For this review, take the finished solid that the model builds, in its own axes (mm). Face numbers are marked on the shaded views. A direction names the side the tool comes from. Coordinates: 2 decimals unless noted, no trailing zeros. Write each loop counter-clockwise with the first axis right and the second up, starting at its lowest first coordinate (ties: lowest second). Pieces come first, ordered by that corner, then holes. Notation, with made-up numbers: (4.25, -11.5) - (20.25, -11.5) arc R22 cw to (20.25, 24.5) - close; hole circle Ø4 at (1, -28.75). An arc over 180 degrees is marked (long way). Write each question's results on one line, items separated by ' | '.
from build123d import *

# Parameters (mm, degrees)
BOSS_EXTRUDE1_DEPTH     = 177.8
BOSS_EXTRUDE2_DEPTH     = 6.35
BOSS_EXTRUDE3_START     = -6.35
BOSS_EXTRUDE3_DEPTH     = 6.35
SKETCH5_W               = 81.82
SKETCH5_H               = 165.1
CUT_EXTRUDE1_DEPTH      = 216.897319711
BOSS_EXTRUDE6_DEPTH     = 165.1
CUT_EXTRUDE2_DEPTH      = 212.237817104
CUT_EXTRUDE2_DEPTH_BACK = 212.237817104
SKETCH9_R               = 1.4605
SKETCH10_R              = 0.2159
CUT_EXTRUDE3_DEPTH      = 212.237817104


with BuildPart() as part:
    # Sketch1 → Boss-Extrude1 (new body)
    with BuildSketch(Plane.XY):
        with BuildLine():
            Line((0, 12.912727148), (-56.568542495, 69.481269642))
            Line((-56.568542495, 69.481269642), (-61.058670555, 64.991141582))
            Line((-61.058670555, 64.991141582), (-4.490128061, 8.422599087))
            ThreePointArc((-4.490128061, 8.422599087), (5.116694028, -14.770321092), (-4.490128061, -37.96324127))
            Line((-4.490128061, -37.96324127), (-58.371664787, -91.844777996))
            Line((-58.371664787, -91.844777996), (-53.881536726, -96.334906057))
            Line((-53.881536726, -96.334906057), (0, -42.453369331))
            ThreePointArc((0, -42.453369331), (11.466694028, -14.770321092), (0, 12.912727148))
        make_face()
    extrude(amount=BOSS_EXTRUDE1_DEPTH)

    # Sketch2 → Boss-Extrude2 (add)
    with BuildSketch(Plane(origin=(0, 0, 0), x_dir=(-1, 0, 0), z_dir=(0, 0, -1))):
        with BuildLine():
            Line((61.058670555, 64.991141582), (58.371664787, -91.844777996))
            Line((58.371664787, -91.844777996), (4.490128061, -37.96324127))
            ThreePointArc((4.490128061, -37.96324127), (-5.116694028, -14.770321092), (4.490128061, 8.422599087))
            Line((4.490128061, 8.422599087), (61.058670555, 64.991141582))
        make_face()
    extrude(amount=-BOSS_EXTRUDE2_DEPTH)

    # Sketch4 → Boss-Extrude3 (add)
    with BuildSketch(Plane.XY.offset(177.8).offset(BOSS_EXTRUDE3_START)):
        with BuildLine():
            Line((-61.058670555, 64.991141582), (-58.371664787, -91.844777996))
            Line((-58.371664787, -91.844777996), (-4.490128061, -37.96324127))
            ThreePointArc((-4.490128061, -37.96324127), (5.116694028, -14.770321092), (-4.490128061, 8.422599087))
            Line((-4.490128061, 8.422599087), (-61.058670555, 64.991141582))
        make_face()
    extrude(amount=BOSS_EXTRUDE3_DEPTH)

    # Sketch5 → Cut-Extrude1 (cut, through all)
    with BuildSketch(Plane(origin=(21.226684665, -21.226684665, 0), x_dir=(0.7071067811865512, 0.7071067811865439, 0), z_dir=(0.7071067811865439, -0.7071067811865512, 0))):
        with Locations((-63.309065338, 88.9)):
            Rectangle(SKETCH5_W, SKETCH5_H)
    extrude(amount=-CUT_EXTRUDE1_DEPTH, mode=Mode.SUBTRACT)

    # Sketch8 → Boss-Extrude6 (add)
    with BuildSketch(Plane.XY.offset(6.35)):
        Polygon((-50.843145831, -78.430564434), (-46.35301777, -82.920692495), (-52.467323164, -94.920692495), (-56.957451225, -90.430564434), align=None)
    extrude(amount=BOSS_EXTRUDE6_DEPTH)

    # Sketch9 → Cut-Extrude2 (cut, two sides: drawn at the far end of the back side and taken through both)
    with BuildSketch(Plane.XY.offset(177.8).offset(-CUT_EXTRUDE2_DEPTH_BACK)):
        with Locations((-56.568542495, 51.5207574)):
            Circle(SKETCH9_R)
        with Locations((-38.608030253, 33.560245158)):
            Circle(SKETCH9_R)
    extrude(amount=CUT_EXTRUDE2_DEPTH + CUT_EXTRUDE2_DEPTH_BACK, mode=Mode.SUBTRACT)

    # Sketch10 → Cut-Extrude3 (cut, through all)
    with BuildSketch(Plane(origin=(0, 0, 0), x_dir=(-1, 0, 0), z_dir=(0, 0, -1))):
        with Locations((49.930224033, -91.305962629)):
            Circle(SKETCH10_R)
        with Locations((35.788088496, -77.163827092)):
            Circle(SKETCH10_R)
        with Locations((21.645952872, -63.021691468)):
            Circle(SKETCH10_R)
        with Locations((7.503817248, -48.879555844)):
            Circle(SKETCH10_R)
        with Locations((-6.638318376, -34.737420221)):
            Circle(SKETCH10_R)
    extrude(amount=-CUT_EXTRUDE3_DEPTH, mode=Mode.SUBTRACT)


solid = part.part
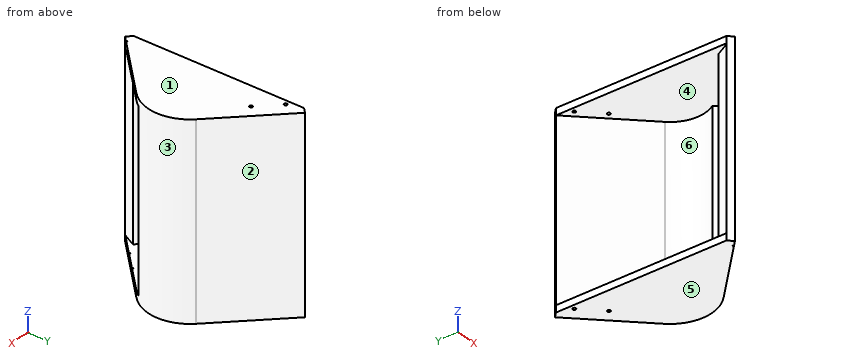
Q1. Mouldability with a two-part tool opening along Y and no side actions: class the marked faces 1, 2, 3 and 4 as pulls with the +Y half, pulls with the -Y half, needs draft (parallel to the pull), parting line crosses it, or undercut.
Results found:
face 1: needs draft | face 2: pulls with the +Y half | face 3: parting line crosses it | face 4: undercut
Q2. Wall thickness on line 1 along Z through (x, y) = (-29.5, -51.5); line 2 along Y through (x, z) = (-49, 49.5): over which ranges is each line inside the solid? List them lowest first. Write a range as from..to.
Results found:
line 1: 0..6.35, 171.45..177.8 | line 2: -88.12..-80.27, 52.93..61.91
Q3. Take a section at A-A on z = 105.5. State the section outline as (x, y) points.
Results found:
outline: (-61.06, 64.99) - (-4.49, 8.42) arc R32.8 cw to (0.26, -31.94) - (4.86, -36.54) arc R39.15 ccw to (0, 12.91) - (-56.57, 69.48) - close; (-58.37, -91.84) - (-53.88, -96.33) - (-52.47, -94.92) - (-46.35, -82.92) - (-50.84, -78.43) - (-56.96, -90.43) - close
Q4. Take a section at C-C on x = -19. State the section outline as (y, z) points, plus the area to 3 significant figures.
Results found:
outline: (-61.45, 0) - (31.91, 0) - (31.91, 177.8) - (-61.45, 177.8) - (-61.45, 171.45) - (22.93, 171.45) - (22.93, 6.35) - (-61.45, 6.35) - close | area: 2,670 mm2
Q5. For pin 1 (10 mm diameter, centred on y = -6.5, z = 44.5, fed in from +X); pin 2 (5 mm diameter, centred on y = 43.5, z = 27.5, fed in from +X); pin 3 (6 mm diameter, centred on x = -26, z = 96.5, fed in from -Y); pin 4 (2.5 mm diameter, centred on x = -38.61, y = 33.56, fed in from -Z), all flat-tipped, find the tip position at first contact; note any pin that passes through.
Results found:
pin 1: x = 11.33 | pin 2: x = -28.09 | pin 3: y = 26.93 | pin 4: through
Q6. Take a section at D-D on y = 16.5. State the section outline as (x, z) points, plus the area to 3 significant figures.
Results found:
outline: (-60.23, 0) - (-3.59, 0) - (-3.59, 177.8) - (-60.23, 177.8) - (-60.23, 171.45) - (-12.57, 171.45) - (-12.57, 6.35) - (-60.23, 6.35) - close | area: 2,200 mm2
Q7. Take a section at B-B on y = -72. State the section outline as (x, z) points, plus the area to 3 significant figures.
Results found:
outline: (-58.71, 0) - (-29.55, 0) - (-29.55, 6.35) - (-58.71, 6.35) - close; (-58.71, 171.45) - (-29.55, 171.45) - (-29.55, 177.8) - (-58.71, 177.8) - close | area: 370 mm2
Q8. For the marked faces 5 and 6, list the 3-axis set-ups (+Z, -Z, +X, -X, +Y, -Y) from which the entire face can be reached by the end or side of a thin tool; tool diameter is ignored.
Results found:
face 5: -Z, +X, -X, +Y, -Y | face 6: -X
